from build123d import *

# Parameters (mm, degrees)
SKETCH1_R           = 4
BOSS_EXTRUDE1_DEPTH = 376
SKETCH2_R           = 1
CUT_EXTRUDE1_DEPTH  = 10
CHAMFER1_SIZE       = 0.5


with BuildPart() as part:
    # Sketch1 → Boss-Extrude1 (new body)
    with BuildSketch(Plane.XY):
        Circle(SKETCH1_R)
    extrude(amount=BOSS_EXTRUDE1_DEPTH)

    # Sketch2 → Cut-Extrude1 (cut)
    with BuildSketch(Plane.XY.offset(376)):
        Circle(SKETCH2_R)
    extrude(amount=-CUT_EXTRUDE1_DEPTH, mode=Mode.SUBTRACT)

    # Chamfer1
    chamfer1_edges = [part.edges().sort_by_distance(p)[0] for p in [
        (-4, 0, 0),
        (-4, 0, 376),
    ]]
    chamfer(chamfer1_edges, length=CHAMFER1_SIZE)


solid = part.part
Check sheet for the modelled part. Datum: model origin and axes. Units: mm. Give positions to 0.01 mm unless a question says otherwise; leave off trailing zeros. Write each loop counter-clockwise with the first axis right and the second up, starting at its lowest first coordinate (ties: lowest second). Pieces come first, ordered by that corner, then holes. Notation, with made-up numbers: (27.5, 61.25) -> (31.5, 61.25) arc R22 cw to (31.5, 83.25) -> close; hole circle Ø10 at (-14.75, 35). An arc over 180 degrees is marked (long way). One line per item, written item: value. Start each with the question number.
Item 1: Draft check along X on faces 1 (the cylindrical face through (-0.867, -3.905, 185.375)), 2 (the flat face through (0, 0, 0)). Enter one of: +X half, -X half, draft (parallel to the pull), parting line (faces both ways), or undercut.
Item 2: Gauge pin test, flat ends, axial feed: pin 1 (0.6 mm diameter, centred on x = 0, y = 0, fed in from +Z); pin 2 (1 mm diameter, centred on x = 2.5, z = 65.5, fed in from -Y). Record the tip position at first contact, or that the pin passes through.
Item 3: Section check A-A on z = 28. Record the cut outline in (x, y).
Item 4: Material ranges on probe 1 along Y at (x, z) = (0, 373.75); probe 2 along Y at (x, z) = (0.25, 355.5); probe 3 along Y at (x, z) = (-2, 49.5), recorded low to high. Write a range as from..to.
Results list:
1. face 1: parting line
1. face 2: draft
2. pin 1: z = 366
2. pin 2: y = -3.46
3. outline: circle Ø8 at (0, 0)
4. probe 1: -4..-1, 1..4
4. probe 2: -3.99..3.99
4. probe 3: -3.46..3.46
